Design review of the part shown in the three views and the two pictorial views. Dimensions are in mm from the part's minimum x, y and z. Coordinates: 2 decimals unless noted, no trailing zeros. Loops run counter-clockwise (first coordinate to the right, second up) from the corner with the lowest first, then second, coordinate; pieces in that order, holes last. Notation, with made-up numbers: M 86.5,-37 L 93.5,-37 A25 ccw 93.5,-22 Z; hole C 51.25,-9 d11. An arc over 180 degrees is marked long. Answer as a JSON object with one key per item and string values. Group by question number.
Item 1: Wall thickness on L1, parallel to Y at x = 132, z = 3.75; L2, parallel to X at y = 59, z = 4.5; L3, parallel to X at y = 42, z = 6: over which ranges is each line inside the solid? List them lowest first. Write a range as from..to.
Item 2: Add section A-A (x = 100). State the section outline as (y, z) points, then the cut area to 3 significant figures.
Item 3: Insertion check: pin 1 (4 mm diameter, centred on x = 75, y = 23, fed in from -Z). The pin has a flat end and moves straight along its axis. Give the tip position at first contact, or say it passes through.
Item 4: Add section D-D (y = 8). State the section outline as (x, z) points, then the cut area to 3 significant figures.
Item 5: Add section C-C (z = 3.5). Count the separate pieces of the cut face and the enclosed holes in it, then the cut area to 3 significant figures.
Item 6: Add section B-B (y = 43). State the section outline as (x, z) points, then the cut area to 3 significant figures.
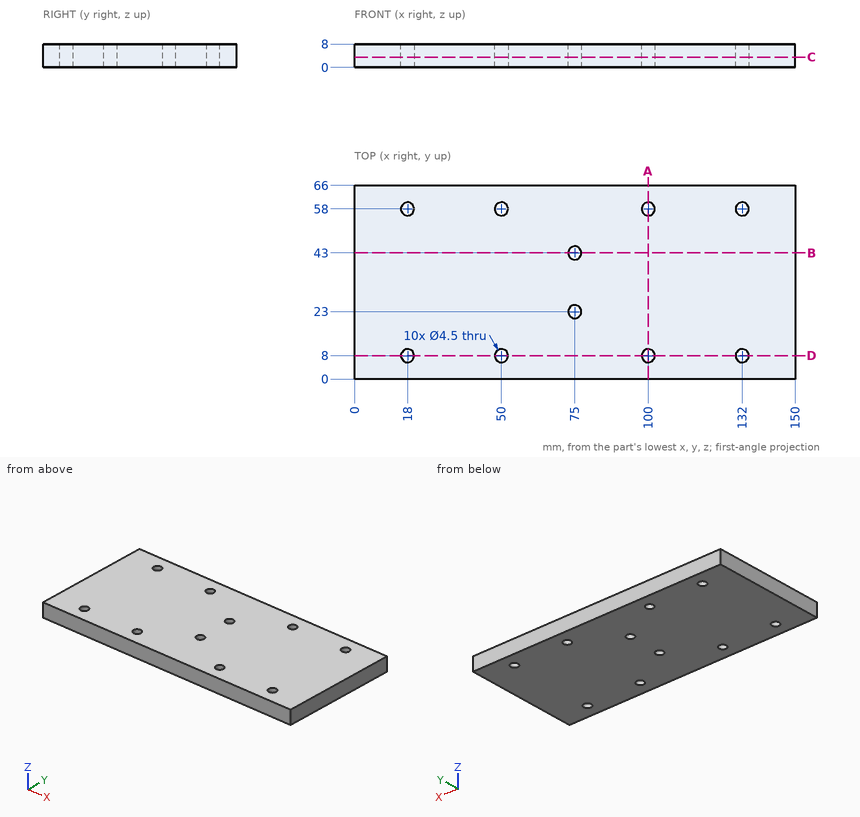
From the geometry:
{
 "1": {"L1": "y = 0..5.75, 10.25..55.75, 60.25..66", "L2": "x = 0..15.98, 20.02..47.98, 52.02..97.98, 102.02..129.98, 134.02..150", "L3": "x = 0..72.98, 77.02..150"},
 "2": {"outline": "M 0,0 L 5.75,0 L 5.75,8 L 0,8 Z; M 10.25,0 L 55.75,0 L 55.75,8 L 10.25,8 Z; M 60.25,0 L 66,0 L 66,8 L 60.25,8 Z", "area": "456 mm²"},
 "3": {"pin 1": "passes through"},
 "4": {"outline": "M 0,0 L 15.75,0 L 15.75,8 L 0,8 Z; M 20.25,0 L 47.75,0 L 47.75,8 L 20.25,8 Z; M 52.25,0 L 97.75,0 L 97.75,8 L 52.25,8 Z; M 102.25,0 L 129.75,0 L 129.75,8 L 102.25,8 Z; M 134.25,0 L 150,0 L 150,8 L 134.25,8 Z", "area": "1,060 mm²"},
 "5": {"separate pieces": "1", "enclosed holes": "10", "area": "9,740 mm²"},
 "6": {"outline": "M 0,0 L 72.75,0 L 72.75,8 L 0,8 Z; M 77.25,0 L 150,0 L 150,8 L 77.25,8 Z", "area": "1,160 mm²"}
}
